```python
from build123d import *

# Parameters (mm, degrees)
ESQUISSE1_R      = 12
EXTRUSION1_DEPTH = 29.2
CONG_1_R         = 1
ESQUISSE2_R      = 4
EXTRUSION2_DEPTH = 24.7
ESQUISSE3_R      = 2
EXTRUSION3_DEPTH = 10


with BuildPart() as part:
    # Esquisse1 → Extrusion1 (new body)
    with BuildSketch(Plane.XY):
        Circle(ESQUISSE1_R)
    extrude(amount=EXTRUSION1_DEPTH)

    # Congé1
    cong_1_edges = [part.edges().sort_by_distance(p)[0] for p in [
        (-12, 0, 29.2),
    ]]
    fillet(cong_1_edges, radius=CONG_1_R)

    # Esquisse2 → Extrusion2 (add)
    with BuildSketch(Plane.XY.offset(29.2)):
        Circle(ESQUISSE2_R)
    extrude(amount=EXTRUSION2_DEPTH)

    # Esquisse3 → Extrusion3 (add)
    with BuildSketch(Plane.XY.offset(53.9)):
        Circle(ESQUISSE3_R)
    extrude(amount=EXTRUSION3_DEPTH)


solid = part.part
```
Geometry: final body of the model. Coordinates: model frame, mm. A direction names the side the tool comes from. Coordinates: 2 decimals unless noted, no trailing zeros. Write each loop counter-clockwise with the first axis right and the second up, starting at its lowest first coordinate (ties: lowest second). Pieces come first, ordered by that corner, then holes. Notation, with made-up numbers: M 52.25,-5.5 L 82.25,-5.5 A18 cw 82.25,22.5 Z; hole C 74.25,35.25 d9. An arc over 180 degrees is marked long. Answer as CSV lines item,"result". Start each with the question number.
Q1. Line query: line 1 (Z direction, x = 1, y = 3.25); line 2 (Z direction, x = 2.75, y = 9.5); line 3 (Y direction, x = -1, z = 55). Output: solid intervals per line, ascending. Write a range as from..to.
Q2. Cut plane C-C on z = 25. Return the cut outline in (x, y).
Q3. Reachability of faces 1 (the flat face through (0, -5, 29.2)), 2 (the cylindrical face through (-11.99, 0.53, 13.9)) from +Z, -Z, +X, -X, +Y, -Y: full face, straight path, thin tool, end or side. Return the list, or none.
Q4. Cut plane A-A on y = 0. Return the cut outline in (x, z), then the cut area to 3 significant figures.
Q5. Pin query (flat end, axial travel): P1, Ø8, axis at y = 5, z = 21.5, coming from the -X side; P2, Ø6, axis at x = -5, y = 1.5, coming from the +Z side; P3, Ø3, axis at x = -6.5, y = -1, coming from the +Z side. Return the tip coordinate at first contact, or that it passes through.
Q6. Cut plane D-D on z = 40.5. Return the cut outline in (x, y), then the cut area to 3 significant figures.
Findings below:
1,line 1,"z = 0..53.9"
1,line 2,"z = 0..29.2"
1,line 3,"y = -1.73..1.73"
2,outline,"C 0,0 d24"
3,face 1,"+Z"
3,face 2,"+Z, -Z"
4,outline,"M -12,0 L 12,0 L 12,28.2 A1 ccw 11,29.2 L 4,29.2 L 4,53.9 L 2,53.9 L 2,63.9 L -2,63.9 L -2,53.9 L -4,53.9 L -4,29.2 L -11,29.2 A1 ccw -12,28.2 Z"
4,area,"938 mm2"
5,P1,"stops at x = -11.96"
5,P2,"stops at z = 53.9"
5,P3,"stops at z = 29.2"
6,outline,"C 0,0 d8"
6,area,"50.3 mm2"
